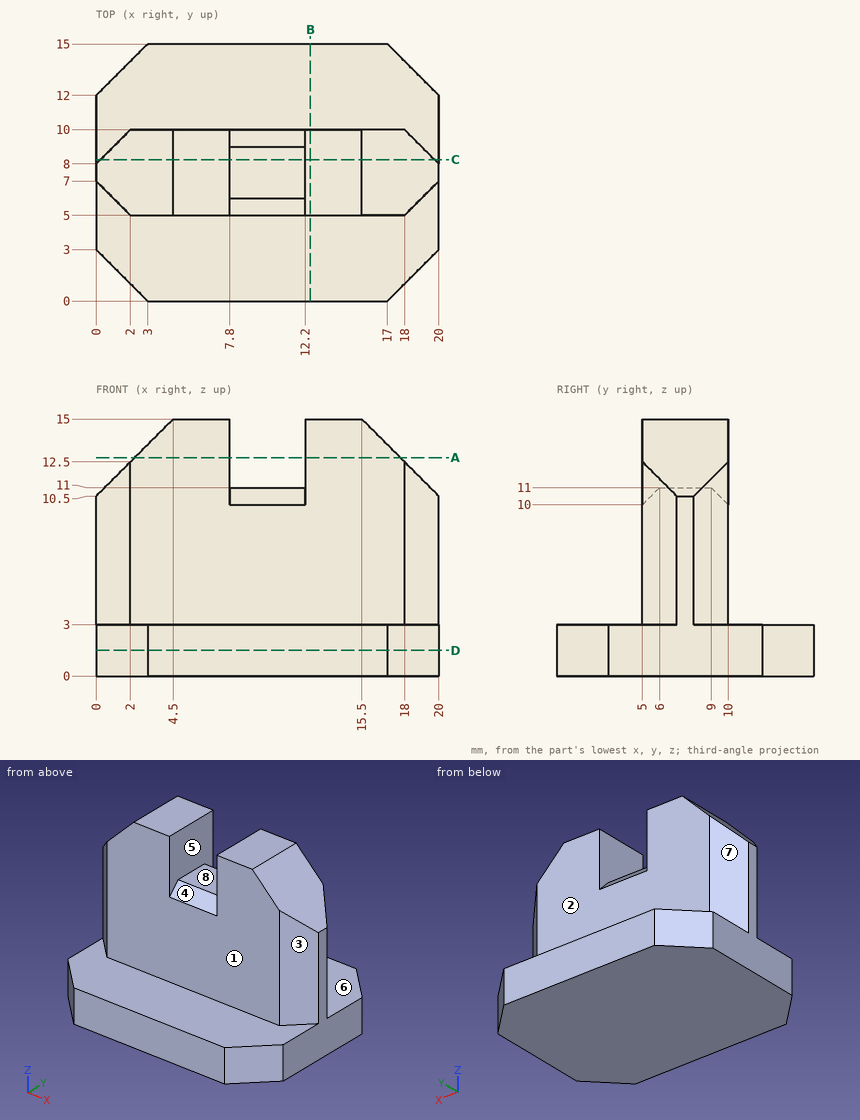
Part print with two shaded views. Sizes in mm from the minimum x, y, z corner. A direction names the side the tool comes from. Give positions to 0.01 mm unless a question says otherwise; leave off trailing zeros. Order: outer loops, then holes, each group sorted by start corner. A loop starts at its lowest first (then second) coordinate and runs counter-clockwise, first axis right, second up.
(1) Saw through at D-D, the plane z = 1.5. Give the cut face in (x, y), then the cut area to 3 significant figures.
(2) Flat gauge pins, fed straight in: pin 1 (1 mm diameter, centred on y = 11.5, z = 10.5, fed in from -X); pin 2 (4 mm diameter, centred on y = 8, z = 13.5, fed in from +X); pin 3 (3 mm diameter, centred on x = 13.5, z = 5.5, fed in from +Y); pin 4 (4 mm diameter, centred on y = 6.5, z = 12.5, fed in from -X). Where does each tip first touch, or does it go through?
(3) Saw through at B-B, the plane x = 12.5. Give the cut face in (y, z).
(4) Tool access for the marked faces 1, 2, 3 and 4: list every direction of +Z, -Z, +X, -X, +Y, -Y with a clear straight run to the whole face (end or side of a thin tool).
(5) Drill centre lines: L1, parallel to X at y = 6.25, z = 12.5; L2, parallel to Y at x = 17.5, z = 6; L3, parallel to Z at x = 3.75, y = 1. Where is each one in solid material? Low to high.
(6) Saw through at C-C, the plane y = 8.25. Give the cut face in (x, z).
(7) Mould opens along X. For the marked faces 5, 6, 7 and 8 say: released by +X, released by -X, zero draft, split by the parting line, or undercut.
(8) Saw through at A-A, the plane z = 12.75. Give the cut face in (x, y).
Results found:
1. outline: (0, 3) - (3, 0) - (17, 0) - (20, 3) - (20, 12) - (17, 15) - (3, 15) - (0, 12) - close
1. area: 282 mm2
2. pin 1: passes through
2. pin 2: stops at x = 19
2. pin 3: stops at y = 10
2. pin 4: stops at x = 0.05
3. outline: (0, 0) - (15, 0) - (15, 3) - (10, 3) - (10, 15) - (5, 15) - (5, 3) - (0, 3) - close
4. face 1: +Z, +X, -X, -Y
4. face 2: +Z, +X, -X, +Y
4. face 3: +Z, +X, -Y
4. face 4: +Z, -Y
5. L1: x = 2 to 7.8, 12.2 to 18
5. L2: y = 5 to 10
5. L3: z = 0 to 3
6. outline: (0, 0) - (20, 0) - (20, 3) - (19.75, 3) - (19.75, 10.75) - (15.5, 15) - (12.2, 15) - (12.2, 11) - (7.8, 11) - (7.8, 15) - (4.5, 15) - (0.25, 10.75) - (0.25, 3) - (0, 3) - close
7. face 5: undercut
7. face 6: zero draft
7. face 7: released by -X
7. face 8: undercut
8. outline: (2.25, 5) - (7.8, 5) - (7.8, 10) - (2.25, 10) - close; (12.2, 5) - (17.75, 5) - (17.75, 10) - (12.2, 10) - close
